Work out the finished part from the listing and answer in its coordinate system (mm). A direction names the side the tool comes from. Give positions to 0.01 mm unless a question says otherwise; leave off trailing zeros. Write each loop counter-clockwise with the first axis right and the second up, starting at its lowest first coordinate (ties: lowest second). Pieces come first, ordered by that corner, then holes. Notation, with made-up numbers: (-23.75, 49.5) -> (34.25, 49.5) arc R27 ccw to (34.25, 82.5) -> close; hole circle Ø5 at (-10, 89.5). An arc over 180 degrees is marked (long way). Write item = value, one per line. Start each with the question number.
from build123d import *

# Parameters (mm, degrees)
F0_W     = 101.6
F0_H     = 50.8
F1_DEPTH = 25.4
F2_R     = 6.35
F3_DEPTH = 25.401
F4_W     = 12.7
F4_H     = 25.4
F6_W     = 8.9851264438
F6_H     = 6.35
F8_R     = 2.53999
F9_SIZE  = 2.54


# Not quite as in the source:
# - a fillet or chamfer is up to 0.001 mm smaller than in the source, because OpenCascade refuses the exact size


with BuildPart() as f1:
    # F0 (on Front) → F1 (new body)
    with BuildSketch(Plane.XZ):
        Rectangle(F0_W, F0_H)
    extrude(amount=F1_DEPTH)

    # F2 (on Front) → F3 (cut, through all)
    with BuildSketch(Plane.XZ):
        with Locations((-38.1, 12.7)):
            Circle(F2_R)
        with Locations((-38.1, -12.7)):
            Circle(F2_R)
        with Locations((38.1, -12.7)):
            Circle(F2_R)
        with Locations((38.1, 12.7)):
            Circle(F2_R)
    extrude(amount=F3_DEPTH, mode=Mode.SUBTRACT)

    # F4 (on Top) → F5 (revolve)
    with BuildSketch(Plane.XY):
        with Locations((6.35, 12.7)):
            Rectangle(F4_W, F4_H)
    revolve(axis=Axis((0, 12.7, 0), (0, 1, 0)))

    # F6 (on Top) → F7 (revolve, cut)
    with BuildSketch(Plane.XY):
        with Locations((-14.6525632219, 13.335)):
            Rectangle(F6_W, F6_H)
    revolve(axis=Axis((0, 6.6735967994, 0), (0, -1, 0)), mode=Mode.SUBTRACT)

    # F8 (radius 2.54 in the source; OpenCascade refuses exactly that, so slightly less here)
    f8_edges = [f1.edges().sort_by_distance(p)[0] for p in [
        (-12.7, 0, 0),
        (10.16, 10.16, 0),
        (-12.7, 16.51, 0),
    ]]
    fillet(f8_edges, radius=F8_R)

    # F9
    f9_edges = [f1.edges().sort_by_distance(p)[0] for p in [
        (0, 0, 25.4),
        (50.8, 0, 0),
        (0, 0, -25.4),
        (-50.8, 0, 0),
    ]]
    chamfer(f9_edges, length=F9_SIZE)


solid = f1.part
(1) Each of these flat-tipped pins is pushed along its axis until it touches: pin 1 (1 mm diameter, centred on y = -2, z = -11, fed in from +X); pin 2 (7.5 mm diameter, centred on x = -38.1, z = -12.7, fed in from +Y); pin 3 (16.5 mm diameter, centred on x = 38.1, z = -12.7, fed in from +Y); pin 4 (8 mm diameter, centred on x = -11.5, y = 3.5, fed in from +Z). Where does it stop, or does it pass through?
(2) Determine the mould class of faces 3 (the flat face through (-49.55, -1.29, -0.36)), 4 (the cylindrical face through (31.756, -12.522, 12.979)), 5 (the flat face through (0, 25.4, 0)) for opening direction X: pulls with the +X half, pulls with the -X half, needs draft (parallel to the pull), parting line crosses it, or undercut.
(3) A cutting plane is placed at D-D, the plane y = 15. Write down the section's boundary in (x, z), then the cut area to 3 significant figures.
(4) For faces 1 (the cylindrical face through (-2.75, 6.4, 12.4)), 2 (the flat face through (-1, -14, 25.4)), determine the directions among +Z, -Z, +X, -X, +Y, -Y from which every point of the face is accessible in a straight line to the end or side of a thin tool.
(5) A cutting plane is placed at B-B, the plane z = -16.5. Write down the section's boundary in (x, y).
(6) A cutting plane is placed at A-A, the plane x = -38.1. Write down the section's boundary in (y, z), then the cut area to 3 significant figures.
(7) Find the intervals of material crossed by line 1 along X through (y, z) = (-18.5, -12.7); line 2 along Z through (x, y) = (38.1, -9.5); line 3 along Z through (x, y) = (36.5, -13), in increasing order.
Results list:
q1.pin_1 = 50.76
q1.pin_2 = through
q1.pin_3 = 0
q1.pin_4 = 23.36
q2.face_3 = pulls with the -X half
q2.face_4 = undercut
q2.face_5 = needs draft
q3.outline = circle Ø20.32 at (0, 0)
q3.area = 324 mm²
q4.face_1 = +Y
q4.face_2 = +Z, +X, -X, +Y, -Y
q5.outline = (-50.8, -25.4) -> (-43.19, -25.4) -> (-43.19, 0) -> (-48.26, 0) -> (-50.8, -2.54) -> close; (-33.01, -25.4) -> (33.01, -25.4) -> (33.01, 0) -> (-33.01, 0) -> close; (43.19, -25.4) -> (50.8, -25.4) -> (50.8, -2.54) -> (48.26, 0) -> (43.19, 0) -> close
q6.outline = (-25.4, -25.4) -> (-2.54, -25.4) -> (0, -22.86) -> (0, -19.05) -> (-25.4, -19.05) -> close; (-25.4, -6.35) -> (0, -6.35) -> (0, 6.35) -> (-25.4, 6.35) -> close; (-25.4, 19.05) -> (0, 19.05) -> (0, 22.86) -> (-2.54, 25.4) -> (-25.4, 25.4) -> close
q6.area = 639 mm²
q7.line_1 = -50.8 to -44.45, -31.75 to 31.75, 44.45 to 50.8
q7.line_2 = -25.4 to -19.05, -6.35 to 6.35, 19.05 to 25.4
q7.line_3 = -25.4 to -18.85, -6.55 to 6.55, 18.85 to 25.4
